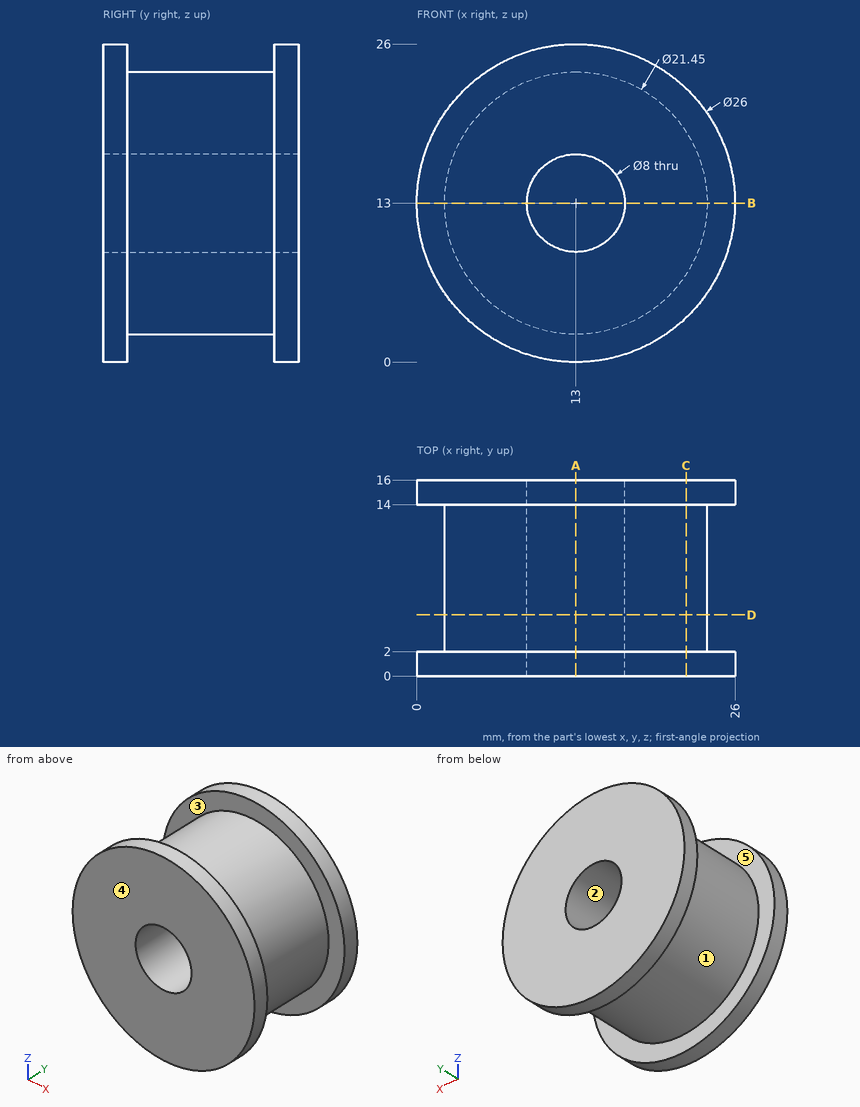
Here's the drawing with two shaded views (mm, measured from the low corner). I have some questions. A direction names the side the tool comes from. Round coordinates to 2 decimals unless told otherwise and drop trailing zeros. Order: outer loops, then holes, each group sorted by start corner. A loop starts at its lowest first (then second) coordinate and runs counter-clockwise, first axis right, second up. Notation, with made-up numbers: (61.5, 33) -> (118.5, 33) arc R13 ccw to (118.5, 45) -> close; hole circle Ø3 at (2, 71.5). An arc over 180 degrees is marked (long way). Use a Markdown table: item, result. Add a question column.
(1) I need wall thicknesses on line 1 along X through (y, z) = (5.5, 12.75); line 2 along Y through (x, z) = (23.75, 12.5); line 3 along X through (y, z) = (12.25, 11.5). Which ranges of each line are inside material? Lowest first, please.
(2) For pin 1 Ø4 at (y, z) = (12.5, 20.5) entering from +X; pin 2 Ø1.5 at (x, y) = (5.5, 11) entering from -Z, each with a flat end and sliding along its axis, tell me the tip position at first contact or that it passes through.
(3) If we mould it in two halves opening along Z, with no side actions, what happens to the marked faces 1, 2 and 3? For each: released by +Z, released by -Z, zero draft, split by the parting line, or undercut.
(4) Suppose I cut it at B-B, the plane z = 13. Please give me the cut outline in (x, y) (3 decimals), and give its area (3 significant figures).
(5) Suppose I cut it at D-D, the plane y = 5. Please give me the cut outline in (x, z) (3 decimals).
(6) Suppose I cut it at C-C, the plane x = 22. Please give me the cut outline in (y, z), and give its area (3 significant figures).
(7) For the marked faces 4 and 5, which set-ups out of +Z, -Z, +X, -X, +Y, -Y let a thin tool reach every point of the face, with its end or its side?
(8) Suppose I cut it at A-A, the plane x = 13. Please give me the cut outline in (y, z) (3 decimals).
Verdict:
| question | item | result |
|---|---|---|
| 1 | line 1 | 2.28 to 9.01, 16.99 to 23.72 |
| 1 | line 2 | 0 to 2, 14 to 16 |
| 1 | line 3 | 2.38 to 9.29, 16.71 to 23.62 |
| 2 | pin 1 | x = 24.44 |
| 2 | pin 2 | z = 4.67 |
| 3 | face 1 | split by the parting line |
| 3 | face 2 | undercut |
| 3 | face 3 | zero draft |
| 4 | outline | (0, 0) -> (9, 0) -> (9, 16) -> (0, 16) -> (0, 14) -> (2.275, 14) -> (2.275, 2) -> (0, 2) -> close; (17, 0) -> (26, 0) -> (26, 2) -> (23.725, 2) -> (23.725, 14) -> (26, 14) -> (26, 16) -> (17, 16) -> close |
| 4 | area | 233 mm2 |
| 5 | outline | circle Ø21.45 at (13, 13); hole circle Ø8 at (13, 13) |
| 6 | outline | (0, 3.62) -> (2, 3.62) -> (2, 7.17) -> (14, 7.17) -> (14, 3.62) -> (16, 3.62) -> (16, 22.38) -> (14, 22.38) -> (14, 18.83) -> (2, 18.83) -> (2, 22.38) -> (0, 22.38) -> close |
| 6 | area | 215 mm2 |
| 7 | face 4 | +Z, -Z, +X, -X, -Y |
| 7 | face 5 | none |
| 8 | outline | (0, 0) -> (2, 0) -> (2, 2.275) -> (14, 2.275) -> (14, 0) -> (16, 0) -> (16, 9) -> (0, 9) -> close; (0, 17) -> (16, 17) -> (16, 26) -> (14, 26) -> (14, 23.725) -> (2, 23.725) -> (2, 26) -> (0, 26) -> close |
